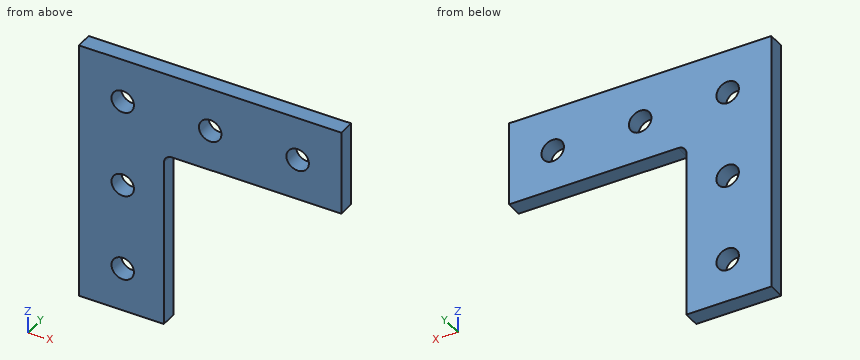
from build123d import *

# Parameters (mm, degrees)
SKETCH1_R      = 3.2639
EXTRUDE1_DEPTH = 4.7752


with BuildPart() as part:
    # Sketch1 → Extrude1 (new body)
    with BuildSketch(Plane(origin=(0, 0, 0), x_dir=(1, 0, 0), z_dir=(0, 1, 0))):
        with BuildLine():
            Line((24.666993976, 76.2), (24.666993976, 27.048243976))
            ThreePointArc((24.666993976, 27.048243976), (25.364445953, 25.364445953), (27.048243976, 24.666993976))
            Line((27.048243976, 24.666993976), (76.2, 24.666993976))
            Line((76.2, 24.666993976), (76.2, 0))
            Line((76.2, 0), (0, 0))
            Line((0, 0), (0, 76.2))
            Line((0, 76.2), (24.666993976, 76.2))
        make_face()
        with Locations(Location((12.7, 63.5, 0), (0, 0, 270))):
            Circle(SKETCH1_R, mode=Mode.SUBTRACT)
        with Locations(Location((12.7, 38.1, 0), (0, 0, 270))):
            Circle(SKETCH1_R, mode=Mode.SUBTRACT)
        with Locations(Location((12.7, 12.7, 0), (0, 0, 270))):
            Circle(SKETCH1_R, mode=Mode.SUBTRACT)
        with Locations(Location((38.1, 12.7, 0), (0, 0, 270))):
            Circle(SKETCH1_R, mode=Mode.SUBTRACT)
        with Locations(Location((63.5, 12.7, 0), (0, 0, 270))):
            Circle(SKETCH1_R, mode=Mode.SUBTRACT)
    extrude(amount=EXTRUDE1_DEPTH)


solid = part.part
Model file for the job. Use its own axes, mm. Coordinates: 2 decimals unless noted, no trailing zeros. Loops run counter-clockwise (first coordinate to the right, second up) from the corner with the lowest first, then second, coordinate; pieces in that order, holes last. Notation, with made-up numbers: (11, 25.25) -> (57, 25.25) arc R33 ccw to (57, 55.25) -> close; hole circle Ø7 at (61, 8.5). An arc over 180 degrees is marked (long way). Use one line per item in the form item = value. Start each with the question number.
(1) Probe probe 1 along X at (y, z) = (1.85, -12.7); probe 2 along X at (y, z) = (3.15, -38.1); probe 3 along X at (y, z) = (2.85, -14.5). List the from-to ranges inside material, lowest first. Write a range as from..to.
(2) Flat gauge pins, fed straight in: pin 1 (2.5 mm diameter, centred on y = 1, z = -43, fed in from +X); pin 2 (2 mm diameter, centred on x = 53, y = 3.5, fed in from -Z). Where does each tip first touch, or does it go through?
(3) Cut at C-C on y = 3.7. Give the cut face in (x, z), and give its area (3 significant figures).
(4) Cut at B-B on z = -38.1. Give the cut face in (x, y).
(5) Cut at A-A on x = 12.7. Give the cut face in (y, z).
(6) Cut at D-D on z = -12.7. Give the cut face in (x, y).
Values:
q1.probe_1 = 0..9.44, 15.96..34.84, 41.36..60.24, 66.76..76.2
q1.probe_2 = 0..9.44, 15.96..24.67
q1.probe_3 = 0..9.98, 15.42..35.38, 40.82..60.78, 66.22..76.2
q2.pin_1 = 24.67
q2.pin_2 = -24.67
q3.outline = (0, -76.2) -> (24.67, -76.2) -> (24.67, -27.05) arc R2.38 cw to (27.05, -24.67) -> (76.2, -24.67) -> (76.2, 0) -> (0, 0) -> close; hole circle Ø6.53 at (12.7, -63.5); hole circle Ø6.53 at (12.7, -38.1); hole circle Ø6.53 at (12.7, -12.7); hole circle Ø6.53 at (38.1, -12.7); hole circle Ø6.53 at (63.5, -12.7)
q3.area = 2,980 mm2
q4.outline = (0, 0) -> (9.44, 0) -> (9.44, 4.78) -> (0, 4.78) -> close; (15.96, 0) -> (24.67, 0) -> (24.67, 4.78) -> (15.96, 4.78) -> close
q5.outline = (0, -76.2) -> (4.78, -76.2) -> (4.78, -66.76) -> (0, -66.76) -> close; (0, -60.24) -> (4.78, -60.24) -> (4.78, -41.36) -> (0, -41.36) -> close; (0, -34.84) -> (4.78, -34.84) -> (4.78, -15.96) -> (0, -15.96) -> close; (0, -9.44) -> (4.78, -9.44) -> (4.78, 0) -> (0, 0) -> close
q6.outline = (0, 0) -> (9.44, 0) -> (9.44, 4.78) -> (0, 4.78) -> close; (15.96, 0) -> (34.84, 0) -> (34.84, 4.78) -> (15.96, 4.78) -> close; (41.36, 0) -> (60.24, 0) -> (60.24, 4.78) -> (41.36, 4.78) -> close; (66.76, 0) -> (76.2, 0) -> (76.2, 4.78) -> (66.76, 4.78) -> close
